For this review, take the finished solid that the model builds, in its own axes (mm). A direction names the side the tool comes from. Round coordinates to 2 decimals unless told otherwise and drop trailing zeros. Order: outer loops, then holes, each group sorted by start corner. A loop starts at its lowest first (then second) coordinate and runs counter-clockwise, first axis right, second up. Notation, with made-up numbers: M 18.25,80.25 L 36.25,80.25 A12 cw 36.25,91.25 Z; hole C 72,65.5 d5. An arc over 180 degrees is marked long. Use a Markdown table: item, result.
from build123d import *

# Parameters (mm, degrees)
F0_R     = 3.25
F1_DEPTH = 15
F2_R     = 1.625
F3_DEPTH = 3
F4_R     = 1


with BuildPart() as f1:
    # F0 (on Top) → F1 (new body)
    with BuildSketch(Plane.XY):
        with BuildLine():
            Line((-4.25, 6.5), (-4.25, 0))
            ThreePointArc((-4.25, 0), (0, -4.25), (4.25, 0))
            Line((4.25, 0), (4.25, 4))
            Line((4.25, 4), (15, 4))
            Line((15, 4), (15, 6.5))
            Line((15, 6.5), (-4.25, 6.5))
        make_face()
        Circle(F0_R, mode=Mode.SUBTRACT)
    extrude(amount=F1_DEPTH)

    # F2 (on face) → F3 (cut)
    with BuildSketch(Plane.XZ.offset(-4)):
        with Locations((9.5, 11)):
            Circle(F2_R)
        with Locations((9.625, 4)):
            Circle(F2_R)
    extrude(amount=-F3_DEPTH, mode=Mode.SUBTRACT)

    # F4
    f4_edges = [f1.edges().sort_by_distance(p)[0] for p in [
        (15, 4, 7.5),
    ]]
    fillet(f4_edges, radius=F4_R)


solid = f1.part
Q1. Draft analysis for pull direction Z (two halves, no side actions). For faces 3 (the cylindrical face through (14.715, 4.301, 7.605)), 4 (the flat face through (3, 4, 15)), 5 (the cylindrical face through (8.21, 5.23, 10.01)), state which applies: pulls with the +Z half, pulls with the -Z half, needs draft (parallel to the pull), parting line crosses it, or undercut.
Determined:
| item | result |
|---|---|
| face 3 | needs draft |
| face 4 | pulls with the +Z half |
| face 5 | undercut |
Q2. Machinability: for faces 1 (the flat face through (4.25, 2, 7)), 2 (the flat face through (6, 6.5, 7)), which of the approach directions +Z, -Z, +X, -X, +Y, -Y give a long, thin tool a straight path to every point of the face, cutting with its end or side? Answer none if there is none.
Determined:
| item | result |
|---|---|
| face 1 | +Z, -Z, +X, -Y |
| face 2 | +Z, -Z, +X, -X, +Y |
Q3. Clearance check with flat-ended pins moving along their axes: pin 1 (1.9 mm diameter, centred on x = 9.625, z = 4, fed in from +Y); pin 2 (1.2 mm diameter, centred on y = 3, z = 5, fed in from +X); pin 3 (1.5 mm diameter, centred on x = 8, z = 12, fed in from -Y); pin 4 (8 mm diameter, centred on x = 7.5, z = 5, fed in from -Y). State where each tip first meets the part, or that it passes through.
Determined:
| item | result |
|---|---|
| pin 1 | passes through |
| pin 2 | stops at x = 4.25 |
| pin 3 | stops at y = 4 |
| pin 4 | stops at y = -2.41 |
Q4. Add section A-A (z = 4). Write out the cut boundary in (x, y).
Determined:
| item | result |
|---|---|
| outline | M -4.25,0 A4.25 ccw 4.25,0 L 4.25,4 L 8,4 L 8,6.5 L -4.25,6.5 Z; M 11.25,4 L 14,4 A1 ccw 15,5 L 15,6.5 L 11.25,6.5 Z; hole C 0,0 d6.5 |
Q5. Add section C-C (y = 1.25). Write out the cut boundary in (x, z), then the cut area to 3 significant figures.
Determined:
| item | result |
|---|---|
| outline | M -4.25,0 L -3,0 L -3,15 L -4.25,15 Z; M 3,0 L 4.25,0 L 4.25,15 L 3,15 Z |
| area | 37.5 mm^2 |
Q6. Wall thickness on line 1 along Z through (x, y) = (9.5, 5.05) (3 decimals); line 2 along Y through (x, z) = (0, 9); line 3 along Z through (x, y) = (9, 5): over which ranges is each line inside the solid? List them lowest first. Write a range as [from, to].
Determined:
| item | result |
|---|---|
| line 1 | z = [0, 2.38], [5.62, 9.375], [12.625, 15] |
| line 2 | y = [-4.25, -3.25], [3.25, 6.5] |
| line 3 | z = [0, 2.5], [5.5, 9.45], [12.55, 15] |
Q7. Add section B-B (x = 0). Write out the cut boundary in (y, z), then the cut area to 4 significant figures.
Determined:
| item | result |
|---|---|
| outline | M -4.25,0 L -3.25,0 L -3.25,15 L -4.25,15 Z; M 3.25,0 L 6.5,0 L 6.5,15 L 3.25,15 Z |
| area | 63.75 mm^2 |
Q8. Add section D-D (x = 9.5). Write out the cut boundary in (y, z) (3 decimals), then the cut area to 3 significant figures.
Determined:
| item | result |
|---|---|
| outline | M 4,0 L 6.5,0 L 6.5,2.38 L 4,2.38 Z; M 4,5.62 L 6.5,5.62 L 6.5,9.375 L 4,9.375 Z; M 4,12.625 L 6.5,12.625 L 6.5,15 L 4,15 Z |
| area | 21.3 mm^2 |
